from build123d import *

# Parameters (mm, degrees)
SKETCH1_R           = 2
BOSS_EXTRUDE1_DEPTH = 3


with BuildPart() as part:
    # Sketch1 → Boss-Extrude1 (new body)
    # profile 1 of 4: a face of its own
    with BuildSketch(Plane(origin=(0, 0, 0), x_dir=(1, 0, 0), z_dir=(0, 1, 0))):
        with BuildLine():
            Line((-30.480543451, -12.568481461), (11.519456549, -12.568481461))
            Line((11.519456549, -12.568481461), (11.519456549, -4.568481461))
            ThreePointArc((11.519456549, -4.568481461), (9.519456549, -4.032583076), (8.055354934, -2.568481461))
            Line((8.055354934, -2.568481461), (-1.016441836, -2.568481461))
            ThreePointArc((-1.016441836, -2.568481461), (-4.480543451, -4.568481461), (-7.944645066, -2.568481461))
            Line((-7.944645066, -2.568481461), (-17.016441836, -2.568481461))
            ThreePointArc((-17.016441836, -2.568481461), (-21.515819631, -4.432184766), (-24.480543451, -0.568481461))
            Line((-24.480543451, -0.568481461), (-26.480543451, -0.568481461))
            ThreePointArc((-26.480543451, -0.568481461), (-28.480543451, -2.568481461), (-30.480543451, -0.568481461))
            Line((-30.480543451, -0.568481461), (-32.480543451, -0.568481461))
            Line((-32.480543451, -0.568481461), (-32.480543451, -10.568481461))
            ThreePointArc((-32.480543451, -10.568481461), (-31.894757013, -11.982695023), (-30.480543451, -12.568481461))
        make_face()
        with Locations(Location((-28.480543451, -8.568481461, 0), (0, 0, 270))):
            Circle(SKETCH1_R, mode=Mode.SUBTRACT)
        with Locations(Location((-20.480543451, -8.568481461, 0), (0, 0, 270))):
            Circle(SKETCH1_R, mode=Mode.SUBTRACT)
        with Locations(Location((-12.480543451, -8.568481461, 0), (0, 0, 270))):
            Circle(SKETCH1_R, mode=Mode.SUBTRACT)
        with Locations(Location((3.519456549, -8.568481461, 0), (0, 0, 270))):
            Circle(SKETCH1_R, mode=Mode.SUBTRACT)
    # profile 2 of 4: a face of its own
    with BuildSketch(Plane(origin=(0, 0, 0), x_dir=(1, 0, 0), z_dir=(0, 1, 0))):
        with BuildLine():
            Line((11.519456549, 3.431518539), (11.519456549, 11.431518539))
            Line((11.519456549, 11.431518539), (-30.480543451, 11.431518539))
            ThreePointArc((-30.480543451, 11.431518539), (-31.894757013, 10.845732102), (-32.480543451, 9.431518539))
            Line((-32.480543451, 9.431518539), (-32.480543451, -0.568481461))
            Line((-32.480543451, -0.568481461), (-30.480543451, -0.568481461))
            ThreePointArc((-30.480543451, -0.568481461), (-28.480543451, 1.431518539), (-26.480543451, -0.568481461))
            Line((-26.480543451, -0.568481461), (-24.480543451, -0.568481461))
            ThreePointArc((-24.480543451, -0.568481461), (-21.515819631, 3.295221845), (-17.016441836, 1.431518539))
            Line((-17.016441836, 1.431518539), (-7.944645066, 1.431518539))
            ThreePointArc((-7.944645066, 1.431518539), (-4.480543451, 3.431518539), (-1.016441836, 1.431518539))
            Line((-1.016441836, 1.431518539), (8.055354934, 1.431518539))
            ThreePointArc((8.055354934, 1.431518539), (9.519456549, 2.895620155), (11.519456549, 3.431518539))
        make_face()
        with Locations(Location((-28.480543451, 7.431518539, 0), (0, 0, 270))):
            Circle(SKETCH1_R, mode=Mode.SUBTRACT)
        with Locations(Location((-20.480543451, 7.431518539, 0), (0, 0, 270))):
            Circle(SKETCH1_R, mode=Mode.SUBTRACT)
        with Locations(Location((-12.480543451, 7.431518539, 0), (0, 0, 270))):
            Circle(SKETCH1_R, mode=Mode.SUBTRACT)
        with Locations(Location((3.519456549, 7.431518539, 0), (0, 0, 270))):
            Circle(SKETCH1_R, mode=Mode.SUBTRACT)
    # profile 3 of 4: a face of its own
    with BuildSketch(Plane(origin=(0, 0, 0), x_dir=(1, 0, 0), z_dir=(0, 1, 0))):
        with BuildLine():
            ThreePointArc((49.519456549, -0.568481461), (51.519456549, 1.431518539), (53.519456549, -0.568481461))
            Line((53.519456549, -0.568481461), (55.519456549, -0.568481461))
            Line((55.519456549, -0.568481461), (55.519456549, 9.431518539))
            ThreePointArc((55.519456549, 9.431518539), (54.933670112, 10.845732102), (53.519456549, 11.431518539))
            Line((53.519456549, 11.431518539), (11.519456549, 11.431518539))
            Line((11.519456549, 11.431518539), (11.519456549, 3.431518539))
            ThreePointArc((11.519456549, 3.431518539), (13.519456549, 2.895620155), (14.983558164, 1.431518539))
            Line((14.983558164, 1.431518539), (24.055354934, 1.431518539))
            ThreePointArc((24.055354934, 1.431518539), (27.519456549, 3.431518539), (30.983558164, 1.431518539))
            Line((30.983558164, 1.431518539), (40.055354934, 1.431518539))
            ThreePointArc((40.055354934, 1.431518539), (44.55473273, 3.295221845), (47.519456549, -0.568481461))
            Line((47.519456549, -0.568481461), (49.519456549, -0.568481461))
        make_face()
        with Locations(Location((19.519456549, 7.431518539, 0), (0, 0, 270))):
            Circle(SKETCH1_R, mode=Mode.SUBTRACT)
        with Locations(Location((35.519456549, 7.431518539, 0), (0, 0, 270))):
            Circle(SKETCH1_R, mode=Mode.SUBTRACT)
        with Locations(Location((43.519456549, 7.431518539, 0), (0, 0, 270))):
            Circle(SKETCH1_R, mode=Mode.SUBTRACT)
        with Locations(Location((51.519456549, 7.431518539, 0), (0, 0, 270))):
            Circle(SKETCH1_R, mode=Mode.SUBTRACT)
    # profile 4 of 4: a face of its own
    with BuildSketch(Plane(origin=(0, 0, 0), x_dir=(1, 0, 0), z_dir=(0, 1, 0))):
        with BuildLine():
            Line((55.519456549, -0.568481461), (53.519456549, -0.568481461))
            ThreePointArc((53.519456549, -0.568481461), (51.519456549, -2.568481461), (49.519456549, -0.568481461))
            Line((49.519456549, -0.568481461), (47.519456549, -0.568481461))
            ThreePointArc((47.519456549, -0.568481461), (44.55473273, -4.432184766), (40.055354934, -2.568481461))
            Line((40.055354934, -2.568481461), (30.983558164, -2.568481461))
            ThreePointArc((30.983558164, -2.568481461), (27.519456549, -4.568481461), (24.055354934, -2.568481461))
            Line((24.055354934, -2.568481461), (14.983558164, -2.568481461))
            ThreePointArc((14.983558164, -2.568481461), (13.519456549, -4.032583076), (11.519456549, -4.568481461))
            Line((11.519456549, -4.568481461), (11.519456549, -12.568481461))
            Line((11.519456549, -12.568481461), (53.519456549, -12.568481461))
            ThreePointArc((53.519456549, -12.568481461), (54.933670112, -11.982695023), (55.519456549, -10.568481461))
            Line((55.519456549, -10.568481461), (55.519456549, -0.568481461))
        make_face()
        with Locations(Location((19.519456549, -8.568481461, 0), (0, 0, 270))):
            Circle(SKETCH1_R, mode=Mode.SUBTRACT)
        with Locations(Location((35.519456549, -8.568481461, 0), (0, 0, 270))):
            Circle(SKETCH1_R, mode=Mode.SUBTRACT)
        with Locations(Location((43.519456549, -8.568481461, 0), (0, 0, 270))):
            Circle(SKETCH1_R, mode=Mode.SUBTRACT)
        with Locations(Location((51.519456549, -8.568481461, 0), (0, 0, 270))):
            Circle(SKETCH1_R, mode=Mode.SUBTRACT)
    extrude(amount=BOSS_EXTRUDE1_DEPTH)


solid = part.part
Here's how the part is built. I have some questions about the finished solid (model axes, mm). A direction names the side the tool comes from. Round coordinates to 2 decimals unless told otherwise and drop trailing zeros. Loops run counter-clockwise (first coordinate to the right, second up) from the corner with the lowest first, then second, coordinate; pieces in that order, holes last. Notation, with made-up numbers: (62.5, -27) -> (90.5, -27) arc R28 cw to (90.5, 4) -> close; hole circle Ø7 at (1.5, 28). An arc over 180 degrees is marked (long way). Write each question's results on one line, items separated by ' | '.
(1) We'd pull the mould along X, two halves only. Please class faces 1 (the face through (11, 3, -5)), 2 (the face through (-30.43, 1.48, 8.13)), 3 (the face through (-31.88, 1.48, -10.86)): released by +X, released by -X, zero draft, split by the parting line, or undercut.
Worked answers:
face 1: zero draft | face 2: undercut | face 3: released by -X
(2) If we section it at D-D, the plane y = 2.15: Give the number of separate pieces and of enclosed holes in the cut face, then the cut area to 3 significant figures.
Worked answers:
separate pieces: 1 | enclosed holes: 19 | area: 1,500 mm2
(3) If I drill on L1, parallel to X at y = 1.3, z = 0.25; L2, parallel to Z at x = -4.5, y = 1.6; L3, parallel to X at y = 2.9, z = -1.5, over which ranges is the centre line in solid material (lowest first)?
Worked answers:
L1: -32.48 to -30.46, -26.51 to -24.47, 47.51 to 49.54, 53.49 to 55.52 | L2: -11.43 to -3.43, 4.57 to 12.57 | L3: -32.48 to -23.9, -17.06 to -7.9, -1.06 to 8.1, 14.94 to 24.1, 30.94 to 40.1, 46.94 to 55.52
(4) If we section it at A-A, the plane x = 36.5: List the corners of the cut face in (y, z) for me.
Worked answers:
outline: (0, -11.43) -> (3, -11.43) -> (3, -9.17) -> (0, -9.17) -> close; (0, -5.69) -> (3, -5.69) -> (3, -1.43) -> (0, -1.43) -> close; (0, 2.57) -> (3, 2.57) -> (3, 6.83) -> (0, 6.83) -> close; (0, 10.31) -> (3, 10.31) -> (3, 12.57) -> (0, 12.57) -> close
(5) For faces 4 (the face through (27.46, 1.48, -3.43)), 5 (the face through (11, 1, 12.568)), which set-ups out of +Z, -Z, +X, -X, +Y, -Y let a thin tool reach every point of the face, with its end or its side?
Worked answers:
face 4: +Y, -Y | face 5: +Z, +X, -X, +Y, -Y
(6) If we section it at C-C, the plane x = 27.5: List the corners of the cut face in (y, z) for me.
Worked answers:
outline: (0, -11.43) -> (3, -11.43) -> (3, -3.43) -> (0, -3.43) -> close; (0, 4.57) -> (3, 4.57) -> (3, 12.57) -> (0, 12.57) -> close
(7) If we section it at B-B, the plane z = -2.25: List the corners of the cut face in (x, y) for me, then the cut area to 3 significant figures.
Worked answers:
outline: (-32.48, 0) -> (-23.32, 0) -> (-23.32, 3) -> (-32.48, 3) -> close; (-17.64, 0) -> (-7.32, 0) -> (-7.32, 3) -> (-17.64, 3) -> close; (-1.64, 0) -> (8.68, 0) -> (8.68, 3) -> (-1.64, 3) -> close; (14.36, 0) -> (24.68, 0) -> (24.68, 3) -> (14.36, 3) -> close; (30.36, 0) -> (40.68, 0) -> (40.68, 3) -> (30.36, 3) -> close; (46.36, 0) -> (55.52, 0) -> (55.52, 3) -> (46.36, 3) -> close | area: 179 mm2
(8) For P1, Ø4.5, axis at x = -28.48, z = 8.57, coming from the -Y side; P2, Ø3.5, axis at x = 19.52, z = -7.43, coming from the +Y side, each with a flat end and sliding along its axis, tell me the tip position at first contact or that it passes through.
Worked answers:
P1: y = 0 | P2: through
